Model file for the job. Use its own axes, mm. Give positions to 0.01 mm unless a question says otherwise; leave off trailing zeros. Loops run counter-clockwise (first coordinate to the right, second up) from the corner with the lowest first, then second, coordinate; pieces in that order, holes last. Notation, with made-up numbers: M 88,22 L 96,22 A28 ccw 96,48 Z; hole C 54,-37.5 d10. An arc over 180 degrees is marked long. Answer in a Markdown table with one row per item.
```python
from build123d import *

# Parameters (mm, degrees)
SKETCH1_W           = 33.02
SKETCH1_H           = 25.4
SKETCH1_R           = 1.651
BOSS_EXTRUDE1_DEPTH = 1.6
SKETCH2_R           = 3.175
SKETCH2_R_2         = 0.4
SKETCH2_R_3         = 1
CUT_EXTRUDE1_DEPTH  = 42.689811705
SKETCH3_R           = 0.508
CUT_EXTRUDE2_DEPTH  = 42.689811705


with BuildPart() as part:
    # Sketch1 → Boss-Extrude1 (new body)
    with BuildSketch(Plane(origin=(0, 0, 0), x_dir=(1, 0, 0), z_dir=(0, 1, 0))):
        with Locations((16.51, 12.7)):
            Rectangle(SKETCH1_W, SKETCH1_H)
        with Locations(Location((5.461, 2.54, 0), (0, 0, 270))):
            Circle(SKETCH1_R, mode=Mode.SUBTRACT)
        with Locations(Location((30.48, 2.54, 0), (0, 0, 270))):
            Circle(SKETCH1_R, mode=Mode.SUBTRACT)
        with Locations(Location((30.48, 22.86, 0), (0, 0, 90))):
            Circle(SKETCH1_R, mode=Mode.SUBTRACT)
        with Locations(Location((5.461, 22.86, 0), (0, 0, 90))):
            Circle(SKETCH1_R, mode=Mode.SUBTRACT)
    extrude(amount=BOSS_EXTRUDE1_DEPTH)

    # Sketch2 → Cut-Extrude1 (cut, through all)
    with BuildSketch(Plane(origin=(0, 1.6, 0), x_dir=(1, 0, 0), z_dir=(0, 1, 0))):
        with Locations(Location((22.78, 12.7, 0), (0, 0, 270))):
            Circle(SKETCH2_R)
        with Locations(Location((27.4, 6.4, 0), (0, 0, 270))):
            Circle(SKETCH2_R_2)
        with Locations(Location((25.4, 6.4, 0), (0, 0, 270))):
            Circle(SKETCH2_R_2)
        with Locations(Location((23.4, 6.4, 0), (0, 0, 270))):
            Circle(SKETCH2_R_2)
        with Locations(Location((21.4, 6.4, 0), (0, 0, 270))):
            Circle(SKETCH2_R_2)
        with Locations(Location((19.4, 6.4, 0), (0, 0, 270))):
            Circle(SKETCH2_R_2)
        with Locations(Location((17.4, 6.4, 0), (0, 0, 270))):
            Circle(SKETCH2_R_2)
        with Locations(Location((15.4, 6.4, 0), (0, 0, 270))):
            Circle(SKETCH2_R_2)
        with Locations(Location((13.4, 6.4, 0), (0, 0, 270))):
            Circle(SKETCH2_R_2)
        with Locations(Location((11.4, 6.4, 0), (0, 0, 270))):
            Circle(SKETCH2_R_2)
        with Locations(Location((9.4, 6.4, 0), (0, 0, 270))):
            Circle(SKETCH2_R_2)
        with Locations(Location((26.4, 19, 0), (0, 0, 270))):
            Circle(SKETCH2_R_2)
        with Locations(Location((24.4, 19, 0), (0, 0, 270))):
            Circle(SKETCH2_R_2)
        with Locations(Location((22.4, 19, 0), (0, 0, 270))):
            Circle(SKETCH2_R_2)
        with Locations(Location((20.4, 19, 0), (0, 0, 270))):
            Circle(SKETCH2_R_2)
        with Locations(Location((18.4, 19, 0), (0, 0, 270))):
            Circle(SKETCH2_R_2)
        with Locations(Location((16.4, 19, 0), (0, 0, 270))):
            Circle(SKETCH2_R_2)
        with Locations(Location((14.4, 19, 0), (0, 0, 270))):
            Circle(SKETCH2_R_2)
        with Locations(Location((12.4, 19, 0), (0, 0, 270))):
            Circle(SKETCH2_R_2)
        with Locations(Location((10.4, 19, 0), (0, 0, 270))):
            Circle(SKETCH2_R_2)
        with Locations(Location((8.4, 19, 0), (0, 0, 270))):
            Circle(SKETCH2_R_2)
        with Locations(Location((22.78, 3.7, 0), (0, 0, 270))):
            Circle(SKETCH2_R_3)
        with Locations(Location((22.78, 21.7, 0), (0, 0, 270))):
            Circle(SKETCH2_R_3)
    extrude(amount=-CUT_EXTRUDE1_DEPTH, mode=Mode.SUBTRACT)

    # Sketch3 → Cut-Extrude2 (cut, through all)
    with BuildSketch(Plane(origin=(0, 1.6, 0), x_dir=(1, 0, 0), z_dir=(0, 1, 0))):
        with Locations(Location((1.27, 1.27, 0), (0, 0, 270))):
            Circle(SKETCH3_R)
        with Locations(Location((1.27, 3.81, 0), (0, 0, 270))):
            Circle(SKETCH3_R)
        with Locations(Location((1.27, 6.35, 0), (0, 0, 270))):
            Circle(SKETCH3_R)
        with Locations(Location((1.27, 8.89, 0), (0, 0, 270))):
            Circle(SKETCH3_R)
        with Locations(Location((1.27, 11.43, 0), (0, 0, 270))):
            Circle(SKETCH3_R)
        with Locations(Location((1.27, 13.97, 0), (0, 0, 270))):
            Circle(SKETCH3_R)
        with Locations(Location((1.27, 16.51, 0), (0, 0, 270))):
            Circle(SKETCH3_R)
        with Locations(Location((1.27, 19.05, 0), (0, 0, 270))):
            Circle(SKETCH3_R)
        with Locations(Location((1.27, 21.59, 0), (0, 0, 270))):
            Circle(SKETCH3_R)
        with Locations(Location((1.27, 24.13, 0), (0, 0, 270))):
            Circle(SKETCH3_R)
    extrude(amount=-CUT_EXTRUDE2_DEPTH, mode=Mode.SUBTRACT)


solid = part.part
```
(1) Saw through at D-D, the plane z = -3.75. Give the cut face in (x, y), and give its area (3 significant figures).
Established:
| item | result |
|---|---|
| outline | M 0,0 L 0.77,0 L 0.77,1.6 L 0,1.6 Z; M 1.77,0 L 4.34,0 L 4.34,1.6 L 1.77,1.6 Z; M 6.58,0 L 21.78,0 L 21.78,1.6 L 6.58,1.6 Z; M 23.78,0 L 29.36,0 L 29.36,1.6 L 23.78,1.6 Z; M 31.6,0 L 33.02,0 L 33.02,1.6 L 31.6,1.6 Z |
| area | 40.8 mm2 |
(2) Saw through at B-B, the plane x = 23.4. Give the cut face in (y, z).
Established:
| item | result |
|---|---|
| outline | M 0,-25.4 L 1.6,-25.4 L 1.6,-22.48 L 0,-22.48 Z; M 0,-20.92 L 1.6,-20.92 L 1.6,-15.81 L 0,-15.81 Z; M 0,-9.59 L 1.6,-9.59 L 1.6,-6.8 L 0,-6.8 Z; M 0,-6 L 1.6,-6 L 1.6,-4.48 L 0,-4.48 Z; M 0,-2.92 L 1.6,-2.92 L 1.6,0 L 0,0 Z |
(3) Mould opens along Z. For faces 1 (the cylindrical face through (21.045, 0.811, -6.215)), 2 (the flat face through (0, 1, -13)), 3 (the flat face through (16, 1, 0)) say: pulls with the +Z half, pulls with the -Z half, needs draft (parallel to the pull), parting line crosses it, or undercut.
Established:
| item | result |
|---|---|
| face 1 | undercut |
| face 2 | needs draft |
| face 3 | pulls with the +Z half |
(4) Wall check: L1, parallel to X at y = 1.1, z = -22.86; L2, parallel to X at y = 0.6, z = -3.81; L3, parallel to Z at x = 29.5, y = 1.2. Give the ranges that are in metal, low to high.
Established:
| item | result |
|---|---|
| L1 | x = 0 to 3.81, 7.11 to 28.83, 32.13 to 33.02 |
| L2 | x = 0 to 0.76, 1.78 to 4.41, 6.52 to 21.79, 23.77 to 29.43, 31.53 to 33.02 |
| L3 | z = -25.4 to -24.19, -21.53 to -3.87, -1.21 to 0 |
(5) Saw through at A-A, the plane x = 30.48. Give the cut face in (y, z), and give its area (3 significant figures).
Established:
| item | result |
|---|---|
| outline | M 0,-25.4 L 1.6,-25.4 L 1.6,-24.51 L 0,-24.51 Z; M 0,-21.21 L 1.6,-21.21 L 1.6,-4.19 L 0,-4.19 Z; M 0,-0.89 L 1.6,-0.89 L 1.6,0 L 0,0 Z |
| area | 30.1 mm2 |
(6) Saw through at C-C, the plane z = -24.13. Give the cut face in (x, y), and give its area (3 significant figures).
Established:
| item | result |
|---|---|
| outline | M 0,0 L 0.76,0 L 0.76,1.6 L 0,1.6 Z; M 1.78,0 L 4.41,0 L 4.41,1.6 L 1.78,1.6 Z; M 6.52,0 L 29.43,0 L 29.43,1.6 L 6.52,1.6 Z; M 31.53,0 L 33.02,0 L 33.02,1.6 L 31.53,1.6 Z |
| area | 44.5 mm2 |
